Input: dimensioned drawing with shaded views. Units: mm. Origin: part minimum x, y, z. A direction names the side the tool comes from. Give positions to 0.01 mm unless a question says otherwise; leave off trailing zeros. Write each loop counter-clockwise with the first axis right and the second up, starting at its lowest first coordinate (ties: lowest second). Pieces come first, ordered by that corner, then holes. Notation, with made-up numbers: (35.5, 4.5) -> (63.5, 4.5) arc R30 ccw to (63.5, 34.5) -> close; hole circle Ø3 at (78, 32.25). An arc over 180 degrees is marked (long way). Answer in a Markdown table with one row per item. Add a question column.
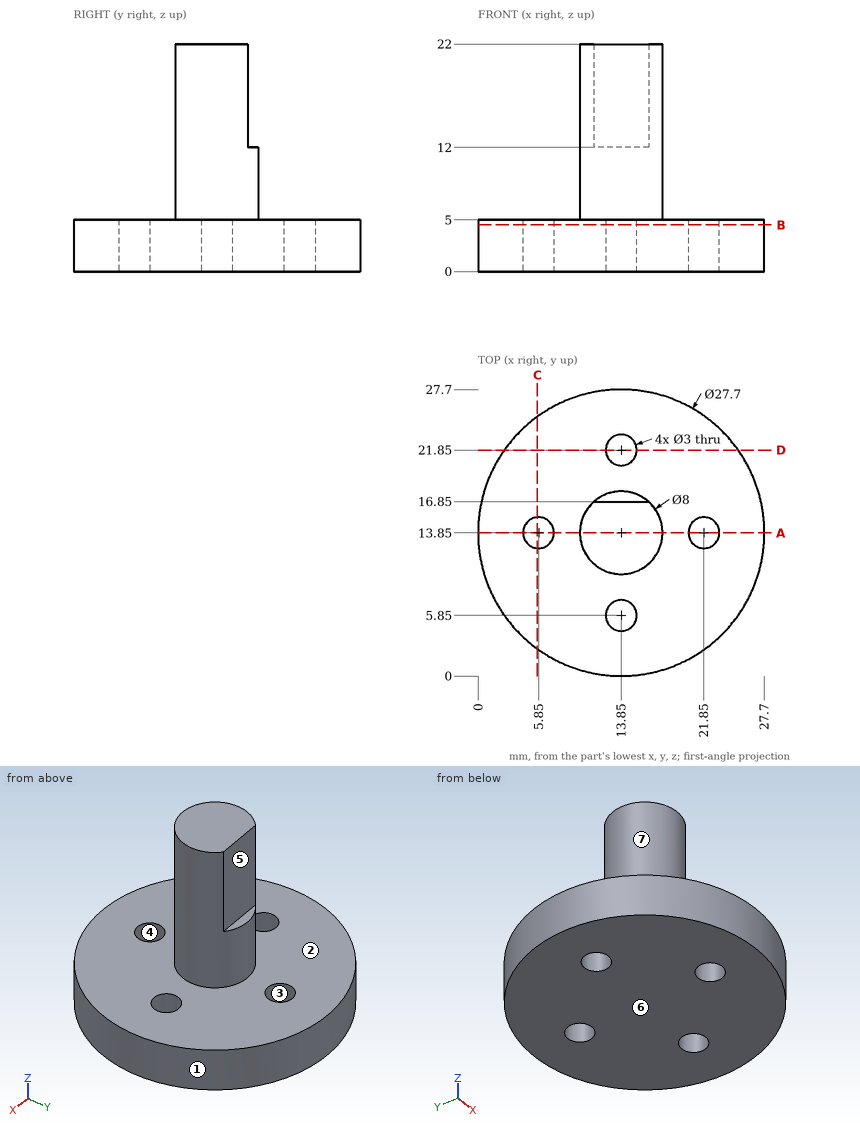
Q1. Line query: probe 1 along Y at (x, z) = (13.85, 2.6); probe 2 along Z at (x, y) = (25, 13.75); probe 3 along Y at (x, z) = (5.85, 3.8). Output: solid intervals per line, ascending. Write a range as from..to.
Q2. Section D-D on y = 21.85. Return loops of the section in (x, z).
Q3. Section C-C on x = 5.75. Return loops of the section in (y, z), and give its area (3 significant figures).
Q4. Section A-A on y = 13.85. Return loops of the section in (x, z).
Q5. Contact query for flat-ended pins moving along their axis: pin 1 Ø1 at (x, y) = (6.5, 21.5) entering from -Z; pin 2 Ø1.6 at (x, z) = (15, 18) entering from +Y; pin 3 Ø1.1 at (x, y) = (13.5, 17.5) entering from +Z; pin 4 Ø12 at (y, z) = (21.5, 12.5) entering from +X. Output: stop coordinate, or through.
Q6. Access query for the marked faces 5, 6 and 7. Directions: +Z, -Z, +X, -X, +Y, -Y. A direction counts if a zero-diameter tool reaches every point of the face in a straight line with its end or side. Return the directions, or none.
Q7. Pull-direction query (X, two-part tool) for the marked faces 1, 2, 3 and 4; classes: +X half, -X half, draft (parallel to the pull), parting line (faces both ways), or undercut.
Q8. Section B-B on z = 4.5. Return loops of the section in (x, y).
Checks:
| question | item | result |
|---|---|---|
| 1 | probe 1 | 0..4.35, 7.35..20.35, 23.35..27.7 |
| 1 | probe 2 | 0..5 |
| 1 | probe 3 | 2.54..12.35, 15.35..25.16 |
| 2 | outline | (2.54, 0) -> (12.35, 0) -> (12.35, 5) -> (2.54, 5) -> close; (15.35, 0) -> (25.16, 0) -> (25.16, 5) -> (15.35, 5) -> close |
| 3 | outline | (2.62, 0) -> (12.35, 0) -> (12.35, 5) -> (2.62, 5) -> close; (15.35, 0) -> (25.08, 0) -> (25.08, 5) -> (15.35, 5) -> close |
| 3 | area | 97.4 mm^2 |
| 4 | outline | (0, 0) -> (4.35, 0) -> (4.35, 5) -> (0, 5) -> close; (7.35, 0) -> (20.35, 0) -> (20.35, 5) -> (17.85, 5) -> (17.85, 22) -> (9.85, 22) -> (9.85, 5) -> (7.35, 5) -> close; (23.35, 0) -> (27.7, 0) -> (27.7, 5) -> (23.35, 5) -> close |
| 5 | pin 1 | z = 0 |
| 5 | pin 2 | y = 16.85 |
| 5 | pin 3 | z = 12 |
| 5 | pin 4 | x = 17.49 |
| 6 | face 5 | +Z, +X, -X, +Y |
| 6 | face 6 | -Z, +X, -X, +Y, -Y |
| 6 | face 7 | +Z |
| 7 | face 1 | parting line |
| 7 | face 2 | draft |
| 7 | face 3 | undercut |
| 7 | face 4 | undercut |
| 8 | outline | circle Ø27.7 at (13.85, 13.85); hole circle Ø3 at (5.85, 13.85); hole circle Ø3 at (13.85, 5.85); hole circle Ø3 at (13.85, 21.85); hole circle Ø3 at (21.85, 13.85) |
